```python
from build123d import *

# Parameters (mm, degrees)
SKETCH1_R           = 14
BOSS_EXTRUDE1_DEPTH = 8
FILLET2_R           = 6
SKETCH2_R           = 2.1
CUT_EXTRUDE1_DEPTH  = 35.365680555
FILLET3_SIZE        = 5
FILLET3_SIZE_2      = 2


with BuildPart() as part:
    # Sketch1 → Boss-Extrude1 (new body)
    with BuildSketch(Plane(origin=(0, 0, 0), x_dir=(1, 0, 0), z_dir=(0, 1, 0))):
        with BuildLine():
            Line((0, -16), (6, -16))
            Line((6, -16), (11, -13))
            Line((11, -13), (26, -13))
            Line((26, -13), (26, -5))
            Line((26, -5), (16, -5))
            Line((16, -5), (16, 0))
            ThreePointArc((16, 0), (-11.313708499, 11.313708499), (0, -16))
        make_face()
        with Locations(Location((0, 0, 0), (0, 0, 270))):
            Circle(SKETCH1_R, mode=Mode.SUBTRACT)
    extrude(amount=BOSS_EXTRUDE1_DEPTH)

    # Fillet2
    fillet2_edges = [part.edges().sort_by_distance(p)[0] for p in [
        (11, 4, 13),
        (6, 4, 16),
    ]]
    fillet(fillet2_edges, radius=FILLET2_R)

    # Sketch2 → Cut-Extrude1 (cut, through all)
    with BuildSketch(Plane(origin=(0, 0, 5), x_dir=(-1, 0, 0), z_dir=(0, 0, -1))):
        with Locations((-22, 4)):
            Circle(SKETCH2_R)
    extrude(amount=-CUT_EXTRUDE1_DEPTH, mode=Mode.SUBTRACT)

    # Fillet3
    # an asymmetric fillet: 5, 2 mm, written as the material it adds along each edge
    with BuildSketch(Plane(origin=(16, 0, 5), x_dir=(0, 0, -1), z_dir=(0, 1, 0))) as fillet3_piece_1:
        with BuildLine():
            Bezier((FILLET3_SIZE, 0), (0, 0), (0, -FILLET3_SIZE_2), weights=[1, 0.707106781, 1])
            Line((0, -FILLET3_SIZE_2), (0, 0))
            Line((0, 0), (FILLET3_SIZE, 0))
        make_face()
    extrude(amount=8)


solid = part.part
```
Geometry: final body of the model. Coordinates: model frame, mm. A direction names the side the tool comes from. Coordinates: 2 decimals unless noted, no trailing zeros. Order: outer loops, then holes, each group sorted by start corner. A loop starts at its lowest first (then second) coordinate and runs counter-clockwise, first axis right, second up. Notation, with made-up numbers: (18.25, 45) -> (33.25, 45) arc R23 ccw to (33.25, 60) -> close; hole circle Ø7 at (-30.75, -26.75). An arc over 180 degrees is marked (long way). Write each question's results on one line, items separated by ' | '. Start each with the question number.
1) Set-up query: faces 4 (the cylindrical face through (-13.67, 3.94, -3.03)), 5 (the flat face through (20, 6, 5)). Return all of +Z, -Z, +X, -X, +Y, -Y with unobstructed straight access to the full face (end or side cutting, diameter ignored); none if empty.
2) Cut plane B-B, the plane z = -8.5. Output: boundary loops of the cut face in (x, y).
3) Cut plane C-C, the plane y = 4. State how many separate pieces and enclosed holes the cut face has, and give its area (3 significant figures).
4) Cut plane A-A, the plane x = 22. Output: boundary loops of the cut face in (y, z).
5) Cut plane D-D, the plane z = 12.5. Output: boundary loops of the cut face in (x, y), and give its area (3 significant figures).
6) First-contact query: pin 1 (4 mm diameter, centred on x = 20.5, y = 2, fed in from -Z); pin 2 (4 mm diameter, centred on x = 13, y = 3.5, fed in from +Z); pin 3 (2.5 mm diameter, centred on x = 20, y = 5.5, fed in from +Z). Flat tips, straight axial feed; report the tip coordinate or a pass-through.
7) Mould query, pull axis Y, two halves, no side actions, for faces 1 (the flat face through (19, 4, 13)), 2 (the flat face through (13, 8, 7)), 3 (the cylindrical face through (19.997, 4.631, 8.944)). Classes: released by +Y, released by -Y, zero draft, split by the parting line, or undercut.
8) Material intervals for line 1 along Z through (x, y) = (-0.5, 7.5); line 2 along Y through (x, z) = (22, 10.25); line 3 along X through (y, z) = (2.25, 0), sorted ascending.
Checks:
1) face 4: +Y, -Y | face 5: -Z, +X, +Y, -Y
2) outline: (-13.56, 0) -> (-11.12, 0) -> (-11.12, 8) -> (-13.56, 8) -> close; (11.12, 0) -> (13.56, 0) -> (13.56, 8) -> (11.12, 8) -> close
3) separate pieces: 2 | enclosed holes: 1 | area: 269 mm^2
4) outline: (0, 5) -> (1.9, 5) -> (1.9, 13) -> (0, 13) -> close; (6.1, 5) -> (8, 5) -> (8, 13) -> (6.1, 13) -> close
5) outline: (-9.99, 0) -> (-6.3, 0) -> (-6.3, 8) -> (-9.99, 8) -> close; (6.3, 0) -> (26, 0) -> (26, 8) -> (6.3, 8) -> close; hole circle Ø4.2 at (22, 4) | area: 173 mm^2
6) pin 1: z = 5 | pin 2: z = 13.23 | pin 3: z = 13
7) face 1: zero draft | face 2: released by +Y | face 3: undercut
8) line 1: -15.99 to -13.99, 13.99 to 15.99 | line 2: 0 to 1.9, 6.1 to 8 | line 3: -16 to -14, 14 to 16
